Check sheet for the modelled part. Datum: model origin and axes. Units: mm. Face numbers are marked on the shaded views. A direction names the side the tool comes from. Give positions to 0.01 mm unless a question says otherwise; leave off trailing zeros. Write each loop counter-clockwise with the first axis right and the second up, starting at its lowest first coordinate (ties: lowest second). Pieces come first, ordered by that corner, then holes. Notation, with made-up numbers: (-16, 78.25) -> (2, 78.25) arc R20 cw to (2, 86.25) -> close; hole circle Ø4 at (33.25, -25.75). An arc over 180 degrees is marked (long way). Return JSON: item names as keys, results as strings.
Autodesk Inventor part; units mm, degrees
ref_plane "YZ Plane" through (0, 0, 0) normal (1, 0, 0) x (0, 1, 0)
ref_plane "XZ Plane" through (0, 0, 0) normal (0, 1, 0) x (-1, 0, 0)
ref_plane "XY Plane" through (0, 0, 0) normal (0, 0, 1) x (1, 0, 0)
sketch "Sketch1" plane through (0, 0, 0) normal (0, 1, 0) x (-1, 0, 0)
  line L0 (10.75, 4.75) -> (-10.75, 4.75) construction
  line L1 (10.75, -4.75) -> (-10.75, -4.75) construction
  line L2 (13.25, 6) -> (13.25, -6)
  line L3 (0, 4.75) -> (0, -4.75) construction
  line L4 (-11.75, 6) -> (-11.75, -6)
  line L5 (-10.75, 4.75) -> (-10.75, -4.75) construction
  line L6 (10.75, 4.75) -> (10.75, -4.75) construction
  line L7 (13.25, 6) -> (-11.75, 6)
  line L8 (13.25, -6) -> (-11.75, -6)
  point P0 (0, 0)
  point P1 (13.25, 0)
  point P2 (0, 0)
  point P3 (0, -4.75)
  point P4 (-11.75, 0)
  dimension "d0" = 9.5
  dimension "d1" = 25
  dimension "d2" = 21.5
  dimension "d3" = 12
  dimension "d4" = 1
extrude "Extrusion1" add sketch "Sketch1" against normal blind 1
sketch "Sketch2" plane through (0, 0, 0) normal (0, 1, 0) x (1, 0, 0)
  line L0 (-10.75, 4.75) -> (10.75, 4.75)
  line L1 (-13.25, 6) -> (11.75, 6)
  line L2 (10.75, 4.75) -> (10.75, -4.75)
  line L3 (10.75, -4.75) -> (-10.75, -4.75)
  line L4 (-10.75, -4.75) -> (-10.75, -6.052)
  line L5 (-10.75, 4.75) -> (-10.75, 6)
  line L6 (-12.25, -6.052) -> (-12.25, 6)
  line L7 (-13.25, 6) -> (-13.25, -6)
  line L8 (-13.25, -6) -> (-13.25, 6)
  line L9 (-13.25, -6) -> (-12.25, -6)
  line L10 (-10.75, -6) -> (11.75, -6)
  line L11 (-13.25, 6) -> (-12.25, 6)
  line L12 (-10.75, 6) -> (11.75, 6)
  line L13 (11.75, 6) -> (11.75, -6)
  line L14 (11.75, -6) -> (11.75, 6)
  point P0 (0, 0)
  dimension "d7" = 1
extrude "Extrusion2" add sketch "Sketch2" along normal blind 2.6
fillet "Fillet1" radius 3 2 edges at (11.75, 0.8, 6) (11.75, 0.8, -6)
fillet "Fillet2" radius 3 2 edges at (-13.25, 0.8, -6) (-13.25, 0.8, 6)
properties part number "HeadphoneThingy"
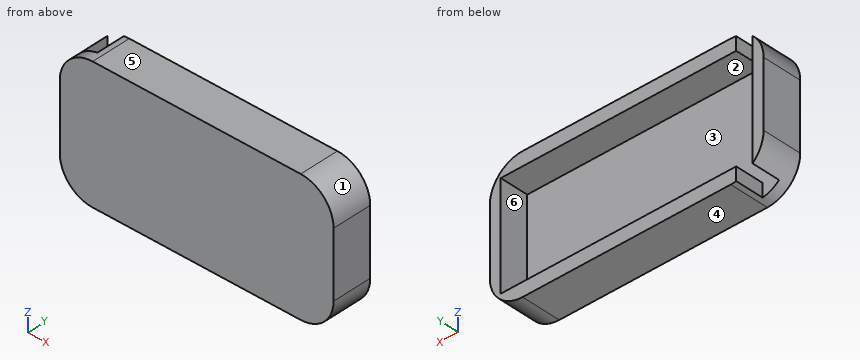
(1) Cross-section at A-A on y = 0.45. Enter the section's corners in (x, z), then the cut area to 3 significant figures.
Reply:
{"outline": "(-13.25, -3) arc R3 ccw to (-12.25, -5.24) -> (-12.25, 5.24) arc R3 ccw to (-13.25, 3) -> close; (-10.75, -5.96) arc R3 ccw to (-10.25, -6) -> (8.75, -6) arc R3 ccw to (11.75, -3) -> (11.75, 3) arc R3 ccw to (8.75, 6) -> (-10.25, 6) arc R3 ccw to (-10.75, 5.96) -> (-10.75, 4.75) -> (10.75, 4.75) -> (10.75, -4.75) -> (-10.75, -4.75) -> close", "area": "71.0 mm^2"}
(2) Cross-section at C-C on x = -8. Enter the section's corners in (y, z).
Reply:
{"outline": "(-1, -6) -> (2.6, -6) -> (2.6, -4.75) -> (0, -4.75) -> (0, 4.75) -> (2.6, 4.75) -> (2.6, 6) -> (-1, 6) -> close"}
(3) Set-up check for the marked faces 1 and 2: record each of +Z, -Z, +X, -X, +Y, -Y from which the full face is reachable in a straight line by a thin tool's end or side.
Reply:
{"face 1": "+Z, +X, +Y, -Y", "face 2": "+Y"}
(4) Depth check by flat-ended pin: pin 1 Ø0.6 at (y, z) = (1.5, -5.5) entering from -X; pin 2 Ø3.5 at (x, z) = (4, -1.5) entering from +Y. Enter the tip coordinate at first touch or a pass-through.
Reply:
{"pin 1": "x = -12.29", "pin 2": "y = 0"}
(5) Release check for a two-part mould opening along Z. For the marked faces 3, 4, 5 and 6 record: pulls with the +Z half, pulls with the -Z half, needs draft (parallel to the pull), parting line crosses it, or undercut.
Reply:
{"face 3": "undercut", "face 4": "pulls with the -Z half", "face 5": "pulls with the +Z half", "face 6": "undercut"}
(6) Thickness scan on L1, parallel to Z at x = -4, y = 0.3; L2, parallel to X at y = 0.15, z = 1.5; L3, parallel to Y at x = -6, z = -4.25. Record the ranges inside material, lowest first.
Reply:
{"L1": "-6 to -4.75, 4.75 to 6", "L2": "-13.25 to -12.25, 10.75 to 11.75", "L3": "-1 to 0"}
(7) Cross-section at D-D on x = -11.25. Enter the section's corners in (y, z), then the cut area to 3 significant figures.
Reply:
{"outline": "(-1, -5.83) -> (0, -5.83) -> (0, 5.83) -> (-1, 5.83) -> close", "area": "11.7 mm^2"}
(8) Cross-section at B-B on z = -0.5. Enter the section's corners in (x, y), then the cut area to 3 significant figures.
Reply:
{"outline": "(-13.25, -1) -> (11.75, -1) -> (11.75, 2.6) -> (10.75, 2.6) -> (10.75, 0) -> (-12.25, 0) -> (-12.25, 2.6) -> (-13.25, 2.6) -> close", "area": "30.2 mm^2"}
